Could you check a few things on this drawing? It's one solid part, dimensions in mm from its lowest x, y, z. Coordinates: 2 decimals unless noted, no trailing zeros. Order: outer loops, then holes, each group sorted by start corner. A loop starts at its lowest first (then second) coordinate and runs counter-clockwise, first axis right, second up.
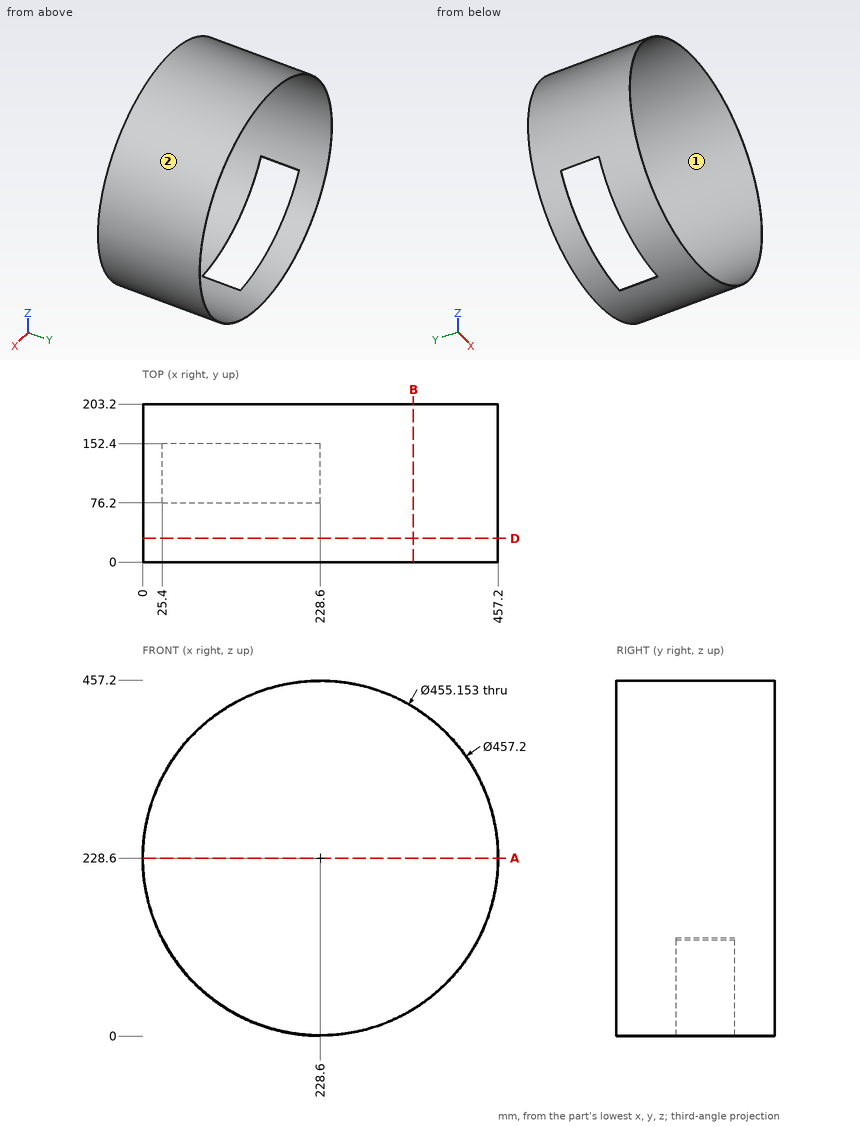
Q1. If we section it at A-A on z = 228.6: Write out the boundary of the cut face in (x, y), then the cut area to 3 significant figures.
Q2. Will these pins go through, and if not, where does the flat tip stop? pin 1 (6 mm diameter, centred on x = 94.5, y = 37, fed in from -Z); pin 2 (1 mm diameter, centred on y = 68, z = 261, fed in from -X); pin 3 (8 mm diameter, centred on y = 159, z = 283, fed in from -X) (3 decimals).
Q3. We'd pull the mould along Z, two halves only. Please class the marked faces 1 and 2: pulls with the +Z half, pulls with the -Z half, needs draft (parallel to the pull), parting line crosses it, or undercut.
Q4. If we section it at D-D on y = 30.5: Write out the boundary of the cut face in (x, z), then the cut area to 3 significant figures.
Q5. I need wall thicknesses on L1, parallel to X at y = 132, z = 228; L2, parallel to Z at x = 222, y = 192.5 (1 decimal). Which ranges of each line are inside material? Lowest first, please.
Q6. If we section it at B-B on x = 348: Write out the boundary of the cut face in (y, z).
Reply:
1. outline: (0, 0) - (1.02, 0) - (1.02, 203.2) - (0, 203.2) - close; (456.18, 0) - (457.2, 0) - (457.2, 203.2) - (456.18, 203.2) - close
1. area: 416 mm2
2. pin 1: stops at z = 41.33
2. pin 2: stops at x = 2.24
2. pin 3: stops at x = 5.625
3. face 1: undercut
3. face 2: parting line crosses it
4. outline: circle Ø457.2 at (228.6, 228.6); hole circle Ø455.15 at (228.6, 228.6)
4. area: 1,470 mm2
5. L1: x = 0 to 1.02, 456.18 to 457.2
5. L2: z = 0.1 to 1.1, 456.1 to 457.1
6. outline: (0, 33.66) - (203.2, 33.66) - (203.2, 34.86) - (0, 34.86) - close; (0, 422.34) - (203.2, 422.34) - (203.2, 423.54) - (0, 423.54) - close
